```python
from build123d import *

# Parameters (mm, degrees)
F0_R     = 2.5
F1_DEPTH = 480


with BuildPart() as f1:
    # F0 (on Top) → F1 (new body)
    with BuildSketch(Plane.XY):
        with BuildLine():
            Line((-154.894894, -55.535871), (-151.894894, -55.535871))
            ThreePointArc((-151.894894, -55.535871), (-150.834234, -55.096531), (-150.394894, -54.035871))
            Line((-150.394894, -54.035871), (-150.394894, -51.035871))
            Line((-150.394894, -51.035871), (-150.394894, -49.135871))
            Line((-150.394894, -49.135871), (-150.694894, -49.135871))
            ThreePointArc((-150.694894, -49.135871), (-150.836316, -49.077292), (-150.894894, -48.935871))
            Line((-150.894894, -48.935871), (-150.894894, -48.635871))
            Line((-150.894894, -48.635871), (-152.194894, -48.635871))
            Line((-152.194894, -48.635871), (-152.194894, -51.035871))
            Line((-152.194894, -51.035871), (-153.834234, -51.035871))
            Line((-153.834234, -51.035871), (-155.909108, -48.960997))
            ThreePointArc((-155.909108, -48.960997), (-156.342654, -48.31215), (-156.494894, -47.546783))
            Line((-156.494894, -47.546783), (-156.494894, -43.524958))
            ThreePointArc((-156.494894, -43.524958), (-156.342654, -42.759591), (-155.909108, -42.110744))
            Line((-155.909108, -42.110744), (-153.834234, -40.035871))
            Line((-153.834234, -40.035871), (-152.194894, -40.035871))
            Line((-152.194894, -40.035871), (-152.194894, -42.435871))
            Line((-152.194894, -42.435871), (-150.894894, -42.435871))
            Line((-150.894894, -42.435871), (-150.894894, -42.135871))
            ThreePointArc((-150.894894, -42.135871), (-150.836316, -41.994449), (-150.694894, -41.935871))
            Line((-150.694894, -41.935871), (-150.394894, -41.935871))
            Line((-150.394894, -41.935871), (-150.394894, -40.035871))
            Line((-150.394894, -40.035871), (-150.394894, -37.035871))
            Line((-150.394894, -37.035871), (-150.394894, -35.535871))
            Line((-150.394894, -35.535871), (-150.394894, -34.035871))
            Line((-150.394894, -34.035871), (-150.394894, -31.035871))
            Line((-150.394894, -31.035871), (-150.394894, -29.135871))
            Line((-150.394894, -29.135871), (-150.694894, -29.135871))
            ThreePointArc((-150.694894, -29.135871), (-150.836316, -29.077292), (-150.894894, -28.935871))
            Line((-150.894894, -28.935871), (-150.894894, -28.635871))
            Line((-150.894894, -28.635871), (-152.194894, -28.635871))
            Line((-152.194894, -28.635871), (-152.194894, -31.035871))
            Line((-152.194894, -31.035871), (-153.834234, -31.035871))
            Line((-153.834234, -31.035871), (-155.909108, -28.960997))
            ThreePointArc((-155.909108, -28.960997), (-156.342654, -28.31215), (-156.494894, -27.546783))
            Line((-156.494894, -27.546783), (-156.494894, -23.524958))
            ThreePointArc((-156.494894, -23.524958), (-156.342654, -22.759591), (-155.909108, -22.110744))
            Line((-155.909108, -22.110744), (-153.834234, -20.035871))
            Line((-153.834234, -20.035871), (-152.194894, -20.035871))
            Line((-152.194894, -20.035871), (-152.194894, -22.435871))
            Line((-152.194894, -22.435871), (-150.894894, -22.435871))
            Line((-150.894894, -22.435871), (-150.894894, -22.135871))
            ThreePointArc((-150.894894, -22.135871), (-150.836316, -21.994449), (-150.694894, -21.935871))
            Line((-150.694894, -21.935871), (-150.394894, -21.935871))
            Line((-150.394894, -21.935871), (-150.394894, -20.035871))
            Line((-150.394894, -20.035871), (-150.394894, -17.035871))
            ThreePointArc((-150.394894, -17.035871), (-150.834234, -15.975211), (-151.894894, -15.535871))
            Line((-151.894894, -15.535871), (-154.894894, -15.535871))
            Line((-154.894894, -15.535871), (-156.294894, -15.535871))
            Line((-156.294894, -15.535871), (-156.794894, -15.535871))
            Line((-156.794894, -15.535871), (-156.794894, -15.835871))
            ThreePointArc((-156.794894, -15.835871), (-156.853473, -15.977292), (-156.994894, -16.035871))
            Line((-156.994894, -16.035871), (-157.294894, -16.035871))
            Line((-157.294894, -16.035871), (-157.294894, -17.335871))
            Line((-157.294894, -17.335871), (-154.894894, -17.335871))
            Line((-154.894894, -17.335871), (-154.894894, -18.975211))
            Line((-154.894894, -18.975211), (-156.969768, -21.050084))
            ThreePointArc((-156.969768, -21.050084), (-157.618615, -21.48363), (-158.383982, -21.635871))
            Line((-158.383982, -21.635871), (-162.405807, -21.635871))
            ThreePointArc((-162.405807, -21.635871), (-163.171174, -21.48363), (-163.820021, -21.050084))
            Line((-163.820021, -21.050084), (-165.894894, -18.975211))
            Line((-165.894894, -18.975211), (-165.894894, -17.335871))
            Line((-165.894894, -17.335871), (-163.494894, -17.335871))
            Line((-163.494894, -17.335871), (-163.494894, -16.035871))
            Line((-163.494894, -16.035871), (-163.794894, -16.035871))
            ThreePointArc((-163.794894, -16.035871), (-163.936316, -15.977292), (-163.994894, -15.835871))
            Line((-163.994894, -15.835871), (-163.994894, -15.535871))
            Line((-163.994894, -15.535871), (-164.494894, -15.535871))
            Line((-164.494894, -15.535871), (-165.894894, -15.535871))
            Line((-165.894894, -15.535871), (-168.894894, -15.535871))
            ThreePointArc((-168.894894, -15.535871), (-169.955555, -15.975211), (-170.394894, -17.035871))
            Line((-170.394894, -17.035871), (-170.394894, -20.035871))
            Line((-170.394894, -20.035871), (-170.394894, -21.935871))
            Line((-170.394894, -21.935871), (-170.094894, -21.935871))
            ThreePointArc((-170.094894, -21.935871), (-169.953473, -21.994449), (-169.894894, -22.135871))
            Line((-169.894894, -22.135871), (-169.894894, -22.435871))
            Line((-169.894894, -22.435871), (-168.594894, -22.435871))
            Line((-168.594894, -22.435871), (-168.594894, -20.035871))
            Line((-168.594894, -20.035871), (-166.955555, -20.035871))
            Line((-166.955555, -20.035871), (-164.880681, -22.110744))
            ThreePointArc((-164.880681, -22.110744), (-164.447135, -22.759591), (-164.294894, -23.524958))
            Line((-164.294894, -23.524958), (-164.294894, -27.546783))
            ThreePointArc((-164.294894, -27.546783), (-164.447135, -28.31215), (-164.880681, -28.960997))
            Line((-164.880681, -28.960997), (-166.955555, -31.035871))
            Line((-166.955555, -31.035871), (-168.594894, -31.035871))
            Line((-168.594894, -31.035871), (-168.594894, -28.635871))
            Line((-168.594894, -28.635871), (-169.894894, -28.635871))
            Line((-169.894894, -28.635871), (-169.894894, -28.935871))
            ThreePointArc((-169.894894, -28.935871), (-169.953473, -29.077292), (-170.094894, -29.135871))
            Line((-170.094894, -29.135871), (-170.394894, -29.135871))
            Line((-170.394894, -29.135871), (-170.394894, -31.035871))
            Line((-170.394894, -31.035871), (-170.394894, -34.035871))
            Line((-170.394894, -34.035871), (-170.394894, -35.535871))
            Line((-170.394894, -35.535871), (-170.394894, -37.035871))
            Line((-170.394894, -37.035871), (-170.394894, -40.035871))
            Line((-170.394894, -40.035871), (-170.394894, -41.935871))
            Line((-170.394894, -41.935871), (-170.094894, -41.935871))
            ThreePointArc((-170.094894, -41.935871), (-169.953473, -41.994449), (-169.894894, -42.135871))
            Line((-169.894894, -42.135871), (-169.894894, -42.435871))
            Line((-169.894894, -42.435871), (-168.594894, -42.435871))
            Line((-168.594894, -42.435871), (-168.594894, -40.035871))
            Line((-168.594894, -40.035871), (-166.955555, -40.035871))
            Line((-166.955555, -40.035871), (-164.880681, -42.110744))
            ThreePointArc((-164.880681, -42.110744), (-164.447135, -42.759591), (-164.294894, -43.524958))
            Line((-164.294894, -43.524958), (-164.294894, -47.546783))
            ThreePointArc((-164.294894, -47.546783), (-164.447135, -48.31215), (-164.880681, -48.960997))
            Line((-164.880681, -48.960997), (-166.955555, -51.035871))
            Line((-166.955555, -51.035871), (-168.594894, -51.035871))
            Line((-168.594894, -51.035871), (-168.594894, -48.635871))
            Line((-168.594894, -48.635871), (-169.894894, -48.635871))
            Line((-169.894894, -48.635871), (-169.894894, -48.935871))
            ThreePointArc((-169.894894, -48.935871), (-169.953473, -49.077292), (-170.094894, -49.135871))
            Line((-170.094894, -49.135871), (-170.394894, -49.135871))
            Line((-170.394894, -49.135871), (-170.394894, -51.035871))
            Line((-170.394894, -51.035871), (-170.394894, -54.035871))
            ThreePointArc((-170.394894, -54.035871), (-169.955555, -55.096531), (-168.894894, -55.535871))
            Line((-168.894894, -55.535871), (-165.894894, -55.535871))
            Line((-165.894894, -55.535871), (-164.494894, -55.535871))
            Line((-164.494894, -55.535871), (-163.994894, -55.535871))
            Line((-163.994894, -55.535871), (-163.994894, -55.235871))
            ThreePointArc((-163.994894, -55.235871), (-163.936316, -55.094449), (-163.794894, -55.035871))
            Line((-163.794894, -55.035871), (-163.494894, -55.035871))
            Line((-163.494894, -55.035871), (-163.494894, -53.735871))
            Line((-163.494894, -53.735871), (-165.894894, -53.735871))
            Line((-165.894894, -53.735871), (-165.894894, -52.096531))
            Line((-165.894894, -52.096531), (-163.820021, -50.021657))
            ThreePointArc((-163.820021, -50.021657), (-163.171174, -49.588112), (-162.405807, -49.435871))
            Line((-162.405807, -49.435871), (-158.383982, -49.435871))
            ThreePointArc((-158.383982, -49.435871), (-157.618615, -49.588112), (-156.969768, -50.021657))
            Line((-156.969768, -50.021657), (-154.894894, -52.096531))
            Line((-154.894894, -52.096531), (-154.894894, -53.735871))
            Line((-154.894894, -53.735871), (-157.294894, -53.735871))
            Line((-157.294894, -53.735871), (-157.294894, -55.035871))
            Line((-157.294894, -55.035871), (-156.994894, -55.035871))
            ThreePointArc((-156.994894, -55.035871), (-156.853473, -55.094449), (-156.794894, -55.235871))
            Line((-156.794894, -55.235871), (-156.794894, -55.535871))
            Line((-156.794894, -55.535871), (-156.294894, -55.535871))
            Line((-156.294894, -55.535871), (-154.894894, -55.535871))
        make_face()
        with Locations((-160.394894, -45.535871)):
            Circle(F0_R, mode=Mode.SUBTRACT)
        with BuildLine():
            ThreePointArc((-156.969768, -41.050084), (-157.618615, -41.48363), (-158.383982, -41.635871))
            Line((-158.383982, -41.635871), (-162.405807, -41.635871))
            ThreePointArc((-162.405807, -41.635871), (-163.171174, -41.48363), (-163.820021, -41.050084))
            Line((-163.820021, -41.050084), (-165.894894, -38.975211))
            Line((-165.894894, -38.975211), (-168.594894, -38.975211))
            Line((-168.594894, -38.975211), (-168.594894, -35.535871))
            Line((-168.594894, -35.535871), (-168.594894, -32.096531))
            Line((-168.594894, -32.096531), (-165.894894, -32.096531))
            Line((-165.894894, -32.096531), (-163.820021, -30.021657))
            ThreePointArc((-163.820021, -30.021657), (-163.171174, -29.588112), (-162.405807, -29.435871))
            Line((-162.405807, -29.435871), (-158.383982, -29.435871))
            ThreePointArc((-158.383982, -29.435871), (-157.618615, -29.588112), (-156.969768, -30.021657))
            Line((-156.969768, -30.021657), (-154.894894, -32.096531))
            Line((-154.894894, -32.096531), (-152.194894, -32.096531))
            Line((-152.194894, -32.096531), (-152.194894, -35.535871))
            Line((-152.194894, -35.535871), (-152.194894, -38.975211))
            Line((-152.194894, -38.975211), (-154.894894, -38.975211))
            Line((-154.894894, -38.975211), (-156.969768, -41.050084))
        make_face(mode=Mode.SUBTRACT)
        with Locations((-160.394894, -25.535871)):
            Circle(F0_R, mode=Mode.SUBTRACT)
    extrude(amount=F1_DEPTH)


solid = f1.part
```
Geometry check sheet. Reference: the model listing, model coordinates, mm. Coordinates: 2 decimals unless noted, no trailing zeros. Use one line per item in the form item = value.
1. Gauge pin test, flat ends, axial feed: pin 1 (1 mm diameter, centred on x = -157.5, z = 241.5, fed in from -Y); pin 2 (1 mm diameter, centred on y = -46.5, z = 49, fed in from -X); pin 3 (4 mm diameter, centred on x = -160.5, z = 282.5, fed in from +Y). Record the tip position at first contact, or that the pin passes through.
Here are the results:
pin_1 = -55.04
pin_2 = -164.29
pin_3 = -21.63
2. Scan lines: line 1 (Y direction, x = -168, z = 118.5); line 2 (X direction, y = -21, z = 120.5); line 3 (Y direction, x = -160.25, z = 371). Record each from-to range of solid material in increasing order.
Here are the results:
line_1 = -55.54 to -51.04, -40.04 to -38.98, -32.1 to -31.04, -20.04 to -15.54
line_2 = -170.39 to -168.59, -165.99 to -163.87, -156.92 to -154.8, -152.19 to -150.39
line_3 = -49.44 to -48.03, -43.04 to -41.64, -29.44 to -28.03, -23.04 to -21.64
3. Section check A-A (z = 169). State how many separate pieces and enclosed holes the cut face has, then the cut area to 3 significant figures.
Here are the results:
separate_pieces = 1
enclosed_holes = 3
area = 292 mm²
